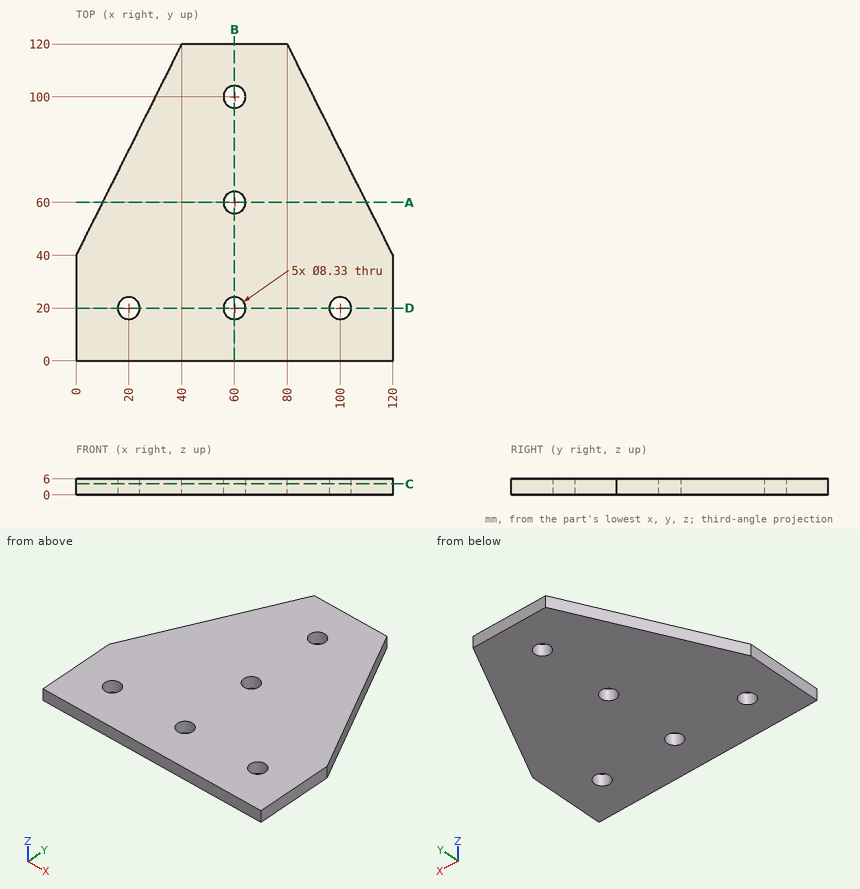
The figure shows three views and two pictorial views of one solid part (mm, origin at its lowest corner). Answer the questions. Round coordinates to 2 decimals unless told otherwise and drop trailing zeros. Loops run counter-clockwise (first coordinate to the right, second up) from the corner with the lowest first, then second, coordinate; pieces in that order, holes last. Notation, with made-up numbers: (64.5, 25) - (81.5, 25) arc R10 cw to (81.5, 44) - close; hole circle Ø4 at (29, 48). An arc over 180 degrees is marked (long way). One line per question, with ' | ' between items. Start each with the question number.
Q1. Find the intervals of material crossed by L1, parallel to Y at x = 60, z = 2.35 (3 decimals); L2, parallel to Y at x = 100, z = 4.1 (3 decimals); L3, parallel to X at y = 61.5, z = 1.85, in increasing order.
Q2. A flat-ended cylindrical pin translates along its axis: pin 1 (1.5 mm diameter, centred on x = 86.5, z = 5.5, fed in from +Y). Find the tip coordinate at first contact, or state that the pin passes through.
Q3. Section A-A on y = 60 is taken. Give the vertices of the cut face in (x, z) (3 decimals), plus the area to 3 significant figures.
Q4. Section B-B on x = 60 is taken. Give the vertices of the cut face in (y, z) (3 decimals), plus the area to 3 significant figures.
Q5. Section C-C on z = 4.15 is taken. Give the vertices of the cut face in (x, y) (3 decimals), plus the area to 3 significant figures.
Established:
1) L1: 0 to 15.835, 24.165 to 55.835, 64.165 to 95.835, 104.165 to 120 | L2: 0 to 15.835, 24.165 to 80 | L3: 10.75 to 56.11, 63.89 to 109.25
2) pin 1: y = 108.5
3) outline: (10, 0) - (55.835, 0) - (55.835, 6) - (10, 6) - close; (64.165, 0) - (110, 0) - (110, 6) - (64.165, 6) - close | area: 550 mm²
4) outline: (0, 0) - (15.835, 0) - (15.835, 6) - (0, 6) - close; (24.165, 0) - (55.835, 0) - (55.835, 6) - (24.165, 6) - close; (64.165, 0) - (95.835, 0) - (95.835, 6) - (64.165, 6) - close; (104.165, 0) - (120, 0) - (120, 6) - (104.165, 6) - close | area: 570 mm²
5) outline: (0, 0) - (120, 0) - (120, 40) - (80, 120) - (40, 120) - (0, 40) - close; hole circle Ø8.33 at (20, 20); hole circle Ø8.33 at (60, 20); hole circle Ø8.33 at (60, 60); hole circle Ø8.33 at (60, 100); hole circle Ø8.33 at (100, 20) | area: 10,900 mm²
